Verification items for the finished model (mm, model axes). A direction names the side the tool comes from. Coordinates: 2 decimals unless noted, no trailing zeros. Write each loop counter-clockwise with the first axis right and the second up, starting at its lowest first coordinate (ties: lowest second). Pieces come first, ordered by that corner, then holes. Notation, with made-up numbers: (71, -11.75) -> (102, -11.75) arc R32 cw to (102, 17.25) -> close; hole circle Ø8 at (45, 21). An arc over 180 degrees is marked (long way). Use CSV: the item, a comma, the result in double quotes.
```python
from build123d import *

# Parameters (mm, degrees)
KES_EKSTR_ZYON1_DEPTH = 1.5


with BuildPart() as part:
    # Çizim1 → Döndür1 (revolve)
    with BuildSketch(Plane.XY):
        Polygon((0, 0), (0, 4), (2.3, 1.7), (11.630773557, 1.7), (11.630773557, 0), align=None)
    revolve(axis=Axis((11.630773557, 0, 0), (-1, 0, 0)))

    # Çizim2 → Kes-Ekstrüzyon1 (cut)
    with BuildSketch(Plane.ZY):
        Polygon((1.154700538, -2), (2.309401077, 0), (1.154700538, 2), (-1.154700538, 2), (-2.309401077, 0), (-1.154700538, -2), align=None)
    extrude(amount=-KES_EKSTR_ZYON1_DEPTH, mode=Mode.SUBTRACT)


solid = part.part
```
1) Gauge pin test, flat ends, axial feed: pin 1 (0.8 mm diameter, centred on x = 0.5, z = 0, fed in from -Y); pin 2 (1.5 mm diameter, centred on x = 9.5, y = -2.5, fed in from -Z); pin 3 (1.5 mm diameter, centred on y = -3, z = 3, fed in from +X); pin 4 (1 mm diameter, centred on x = 4.5, y = 0.5, fed in from +Z). Record the tip position at first contact, or that the pin passes through.
Return value:
pin 1,"y = -3.9"
pin 2,"through"
pin 3,"x = 0.51"
pin 4,"z = 1.7"
2) Scan lines: L1, parallel to X at y = 1, z = -0.75; L2, parallel to X at y = 0, z = 2; L3, parallel to Z at x = 8.5, y = 1.5. Record each from-to range of solid material in increasing order.
Return value:
L1,"1.5 to 11.63"
L2,"1.5 to 2"
L3,"-0.8 to 0.8"
3) Mould release check, pull along Z, two halves, no side actions. Record for faces 3 (the flat face through (1, -2, 0)), 4 (the flat face through (0, -1, -2)), 5 (the cylindrical face through (7.03, -0.37, 1.66)), 6 (the flat face through (0.74, 1.014, -1.724)): released by +Z, released by -Z, zero draft, split by the parting line, or undercut.
Return value:
face 3,"undercut"
face 4,"zero draft"
face 5,"split by the parting line"
face 6,"undercut"
4) Set-up check for faces 1 (the flat face through (1, 2, 0)), 2 (the flat face through (11.631, 0, 0)): record each of +Z, -Z, +X, -X, +Y, -Y from which the full face is reachable in a straight line by a thin tool's end or side.
Return value:
face 1,"-X"
face 2,"+Z, -Z, +X, +Y, -Y"
5) Cross-section at B-B (x = 8.5). Record the boundary of the cut face in (y, z).
Return value:
outline,"circle Ø3.4 at (0, 0)"
6) Cross-section at A-A (z = 0). Record the boundary of the cut face in (x, y), plus the area to 3 significant figures.
Return value:
outline,"(0, -4) -> (2.3, -1.7) -> (11.63, -1.7) -> (11.63, 1.7) -> (2.3, 1.7) -> (0, 4) -> (0, 2) -> (1.5, 2) -> (1.5, -2) -> (0, -2) -> close"
area,"38.8 mm2"
